Verification items for the finished model (mm, model axes). A direction names the side the tool comes from. Give positions to 0.01 mm unless a question says otherwise; leave off trailing zeros. Order: outer loops, then holes, each group sorted by start corner. A loop starts at its lowest first (then second) coordinate and runs counter-clockwise, first axis right, second up.
(1) Scan lines: L1, parallel to Z at x = 37, y = -14.5; L2, parallel to Y at x = 37, z = 2; L3, parallel to X at y = 32.5, z = 7. Record each from-to range of solid material in increasing order.
(2) Gauge pin test, flat ends, axial feed: pin 1 (2.5 mm diameter, centred on y = 24.5, z = 4, fed in from +X); pin 2 (2 mm diameter, centred on x = 35, y = 21.5, fed in from +Z) (3 decimals); pin 3 (4 mm diameter, centred on x = 37, z = 5, fed in from -Y); pin 4 (3.5 mm diameter, centred on y = 37, z = 5, fed in from +X). Record the tip position at first contact, or that the pin passes through.
(3) Sectioned sample at B-B on y = 37. Record the cut outline in (x, z), plus the area to 3 significant figures.
(4) Sectioned sample at D-D on y = -21. Record the cut outline in (x, z), plus the area to 3 significant figures.
(5) Access from +Z, -Z, +X, -X, +Y, -Y to the whole of each face (thin tool, end or side, straight path). Record for faces 1 (the face through (35, 19.233, 5)), 2 (the face through (35, -17.793, 5)), 3 (the face through (0, -30, 5)), 4 (the face through (35, -9.051, 5)).
(6) Sectioned sample at A-A on x = 37. Record the cut outline in (y, z), plus the area to 3 significant figures.
(7) Mould release check, pull along Y, two halves, no side actions. Record for faces 5 (the face through (30, 0, 5)), 6 (the face through (-29, 29, 5)), 7 (the face through (35.8, 13.8, 5.9)): pulls with the +Y half, pulls with the -Y half, needs draft (parallel to the pull), parting line crosses it, or undercut.
(8) Sectioned sample at C-C on z = 1.5. Record the cut outline in (x, y).
Autodesk Inventor part; units mm, degrees
ref_plane "YZ Plane" through (0, 0, 0) normal (1, 0, 0) x (0, 1, 0)
ref_plane "XZ Plane" through (0, 0, 0) normal (0, 1, 0) x (-1, 0, 0)
ref_plane "XY Plane" through (0, 0, 0) normal (0, 0, 1) x (1, 0, 0)
ref_plane "Work Plane1" through (0, 0, 0) normal (0, 0, 1) x (1, 0, 0)
sketch "Sketch1" plane through (0, 0, 0) normal (0, 0, 1) x (1, 0, 0)
  circle A0 centre (17.5, 17.5) radius 1.95
  circle A1 centre (17.5, -17.5) radius 1.95
  circle A2 centre (-17.5, -17.5) radius 1.95
  circle A3 centre (-17.5, 17.5) radius 1.95
  circle A4 centre (0, 0) radius 7.5
  line L0 (-30, 28) -> (-28, 30)
  line L1 (-30, -28) -> (-30, 28)
  line L2 (-28, -30) -> (-30, -28)
  line L3 (28, -30) -> (-28, -30)
  line L4 (30, -28) -> (28, -30)
  line L5 (30, 28) -> (30, -28)
  line L6 (28, 30) -> (30, 28)
  line L7 (-28, 30) -> (28, 30)
extrude "Extrusion1" add sketch "Sketch1" along normal blind 10 contours A0 | A1 | A2 | A3 | A4 | L0 L7 L6 L5 L4 L3 L2 L1
sketch "Sketch2" plane through (0, 0, 10) normal (0, 0, 1) x (1, 0, 0)
  point P0 (0, 0)
sketch "Sketch3" plane through (30, -28, 0) normal (1, 0, 0) x (0, 0, -1)
  line L0 (0, 56) -> (0, 0)
  line L1 (0, 56) -> (-10, 56)
  line L2 (-10, 0) -> (-10, 56)
  line L3 (0, 0) -> (-10, 0)
  line L4 (-10, 0) -> (-10, 56)
  line L5 (0, 47.2331) -> (-10, 47.2331)
  line L6 (-10, 47.2331) -> (-10, 36.3051)
  line L7 (-10, 36.3051) -> (0, 36.3051)
  line L8 (0, 36.3051) -> (0, 47.2331)
  line L9 (0, 56) -> (0, 0)
  line L10 (0, 10.2066) -> (-10, 10.2066)
  line L11 (-10, 10.2066) -> (-10, 18.9489)
  line L12 (-10, 18.9489) -> (0, 18.9489)
  line L13 (0, 18.9489) -> (0, 10.2066)
  point P0 (0, 28)
extrude "Extrusion2" add sketch "Sketch3" along normal blind 14 contours L0 L7 L2 L5 | L0 L10 L2 L12
sketch "Sketch4" plane through (30, 19.2331, 10) normal (0, 1, 0) x (1, 0, 0)
  line L0 (0, 0) -> (0, 10)
  line L1 (0, 0) -> (14, 0)
  line L2 (14, 10) -> (14, 0)
  line L3 (0, 10) -> (14, 10)
  circle A0 centre (7, 5) radius 1.5
  point P0 (-30, 10)
  dimension "d4" = 3
extrude "Extrusion3" cut sketch "Sketch4" against normal through all contours A0
pattern_circular "Circular Pattern1" count 2 over 90 about axis through (0, 0, 0) along (0, 0, 1) of "Extrusion2", "Extrusion3"
properties part number "00_XY_stage-CHUO_SEIKI_LD-647-R1-Middle"
Ans:
1. L1: z = 0 to 3.5, 6.5 to 10
1. L2: y = -17.79 to -9.05, 8.31 to 19.23
1. L3: x = -19.23 to -8.31, 9.05 to 17.79
2. pin 1: stops at x = 30
2. pin 2: passes through
2. pin 3: stops at y = -17.79
2. pin 4: stops at x = 17.79
3. outline: (-19.23, 0) - (-8.31, 0) - (-8.31, 3.5) - (-19.23, 3.5) - close; (-19.23, 6.5) - (-8.31, 6.5) - (-8.31, 10) - (-19.23, 10) - close; (9.05, 0) - (17.79, 0) - (17.79, 3.5) - (9.05, 3.5) - close; (9.05, 6.5) - (17.79, 6.5) - (17.79, 10) - (9.05, 10) - close
3. area: 138 mm2
4. outline: (-30, 0) - (30, 0) - (30, 10) - (-30, 10) - close
4. area: 600 mm2
5. face 1: +Z, -Z, +X, +Y
5. face 2: +Z, -Z, +X, -Y
5. face 3: +Z, -Z, +X, -X, -Y
5. face 4: +Z, -Z, +X
6. outline: (-17.79, 0) - (-9.05, 0) - (-9.05, 3.5) - (-17.79, 3.5) - close; (-17.79, 6.5) - (-9.05, 6.5) - (-9.05, 10) - (-17.79, 10) - close; (8.31, 0) - (19.23, 0) - (19.23, 3.5) - (8.31, 3.5) - close; (8.31, 6.5) - (19.23, 6.5) - (19.23, 10) - (8.31, 10) - close
6. area: 138 mm2
7. face 5: undercut
7. face 6: pulls with the +Y half
7. face 7: needs draft
8. outline: (-30, -28) - (-28, -30) - (28, -30) - (30, -28) - (30, -17.79) - (44, -17.79) - (44, -9.05) - (30, -9.05) - (30, 8.31) - (44, 8.31) - (44, 19.23) - (30, 19.23) - (30, 28) - (28, 30) - (17.79, 30) - (17.79, 44) - (9.05, 44) - (9.05, 30) - (-8.31, 30) - (-8.31, 44) - (-19.23, 44) - (-19.23, 30) - (-28, 30) - (-30, 28) - close
